Autodesk Inventor part; units mm, degrees
ref_plane "YZ Plane" through (0, 0, 0) normal (1, 0, 0) x (0, 1, 0)
ref_plane "XZ Plane" through (0, 0, 0) normal (0, 1, 0) x (-1, 0, 0)
ref_plane "XY Plane" through (0, 0, 0) normal (0, 0, 1) x (1, 0, 0)
sketch "Sketch1" plane through (0, 0, 0) normal (0, 0, 1) x (1, 0, 0)
  line L0 (-12.121, 12.2642) -> (187.879, 12.2642)
  line L1 (187.879, 12.2642) -> (187.879, -187.7358)
  line L2 (187.879, -187.7358) -> (-12.121, -187.7358)
  line L3 (-12.121, -187.7358) -> (-12.121, 12.2642)
  point P0 (0, 0)
  dimension "d0" = 200
  dimension "d1" = 200
  dimension "d2" = 200
extrude "Extrusion1" add sketch "Sketch1" along normal blind 3
sketch "Sketch2" plane through (0, 0, 3) normal (0, 0, 1) x (1, 0, 0)
  circle A0 centre (30.5932, -28.4894) radius 2.0324
  line L0 (187.879, -187.7358) -> (187.879, 12.2642)
  circle A1 centre (145.0597, -28.4894) radius 2.0324
  line L1 (62.879, -127.7358) -> (112.879, -127.7358)
  line L2 (112.879, -127.7358) -> (112.879, -157.7358)
  line L3 (112.879, -157.7358) -> (62.879, -157.7358)
  line L4 (62.879, -157.7358) -> (62.879, -127.7358)
  line L5 (-12.121, -187.7358) -> (187.879, -187.7358)
  line L6 (-12.121, 12.2642) -> (-12.121, -187.7358)
  point P0 (0, 0)
  point P1 (42.5932, -63.9945)
  point P2 (133.0597, -63.9945)
  point P3 (62.879, -142.7358)
  dimension "d14" = 12
  dimension "d15" = 12
  dimension "d16" = 50
  dimension "d17" = 30
  dimension "d18" = 30
  dimension "d19" = 75
extrude "Extrusion2" cut sketch "Sketch2" against normal blind 3
properties part number "facef" material "Glass"
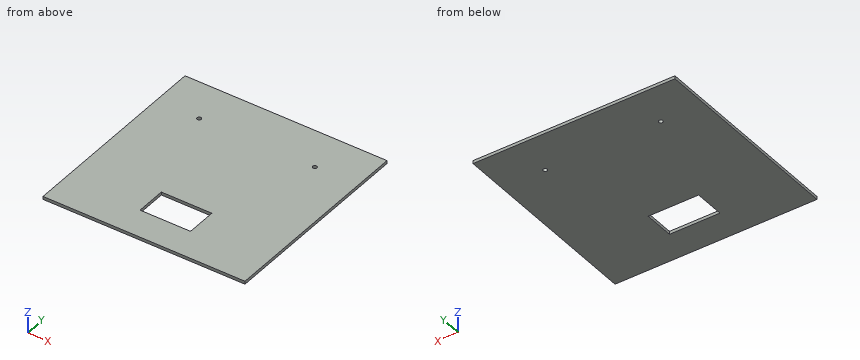
Could you check a few things on this model? Use its own coordinates, in mm. Give positions to 0.01 mm unless a question says otherwise; leave off trailing zeros. Order: outer loops, then holes, each group sorted by start corner. A loop starts at its lowest first (then second) coordinate and runs counter-clockwise, first axis right, second up.
1. Suppose I cut it at A-A (y = -136). List the corners of the cut face in (x, z) for me, plus the area to 3 significant figures.
2. Suppose I cut it at C-C (z = 1.3). List the corners of the cut face in (x, y) for me, plus the area to 3 significant figures.
3. I need wall thicknesses on L1, parallel to X at y = -133, z = 2.05; L2, parallel to Y at x = 90, z = 0.6. Which ranges of each line are inside material? Lowest first, please.
4. Will these pins go through, and if not, where does the flat tip stop? P1, Ø5.5, axis at x = 145.06, y = -28.49, coming from the +Z side; P2, Ø3.5, axis at x = 30.59, y = -28.49, coming from the -Z side.
5. Suppose I cut it at B-B (x = 83). List the corners of the cut face in (y, z) for me.
Solved:
1. outline: (-12.12, 0) - (62.88, 0) - (62.88, 3) - (-12.12, 3) - close; (112.88, 0) - (187.88, 0) - (187.88, 3) - (112.88, 3) - close
1. area: 450 mm2
2. outline: (-12.12, -187.74) - (187.88, -187.74) - (187.88, 12.26) - (-12.12, 12.26) - close; hole circle Ø4.06 at (30.59, -28.49); hole (62.88, -157.74) - (112.88, -157.74) - (112.88, -127.74) - (62.88, -127.74) - close; hole circle Ø4.06 at (145.06, -28.49)
2. area: 38,500 mm2
3. L1: x = -12.12 to 62.88, 112.88 to 187.88
3. L2: y = -187.74 to -157.74, -127.74 to 12.26
4. P1: stops at z = 3
4. P2: passes through
5. outline: (-187.74, 0) - (-157.74, 0) - (-157.74, 3) - (-187.74, 3) - close; (-127.74, 0) - (12.26, 0) - (12.26, 3) - (-127.74, 3) - close
